For this review, use the dimensioned drawing (mm, ordinates from the lowest corner) and the shaded views. A direction names the side the tool comes from. Give positions to 0.01 mm unless a question says otherwise; leave off trailing zeros. Loops run counter-clockwise (first coordinate to the right, second up) from the corner with the lowest first, then second, coordinate; pieces in that order, holes last. Notation, with made-up numbers: (82, 5.25) - (110, 5.25) arc R24 ccw to (110, 20.25) - close; hole circle Ø3 at (45.25, 62.5). An arc over 180 degrees is marked (long way). Write each question's results on one line, items separated by ' | '.
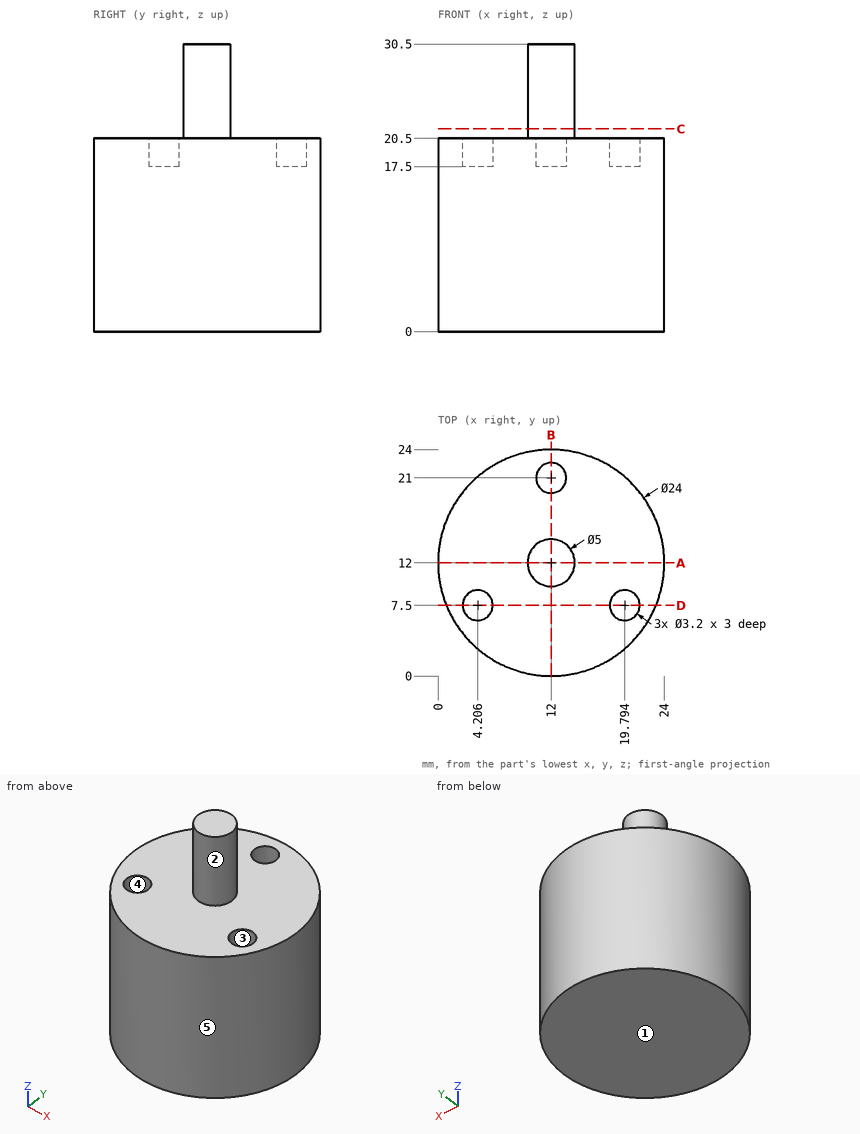
Item 1: We need section B-B on x = 12. Give the boundary of the cut face in (y, z).
Output values:
outline: (0, 0) - (24, 0) - (24, 20.5) - (22.6, 20.5) - (22.6, 17.5) - (19.4, 17.5) - (19.4, 20.5) - (14.5, 20.5) - (14.5, 30.5) - (9.5, 30.5) - (9.5, 20.5) - (0, 20.5) - close
Item 2: Wall thickness on probe 1 along Y at (x, z) = (12, 19.6); probe 2 along Z at (x, y) = (14.5, 7); probe 3 along Y at (x, z) = (6.25, 14): over which ranges is each line inside the solid? List them lowest first.
Output values:
probe 1: y = 0 to 19.4, 22.6 to 24 | probe 2: z = 0 to 20.5 | probe 3: y = 1.47 to 22.53
Item 3: Draft analysis for pull direction Y (two halves, no side actions). For the marked faces 1, 2 and 3, state which applies: +Y half, -Y half, draft (parallel to the pull), parting line (faces both ways), or undercut.
Output values:
face 1: draft | face 2: parting line | face 3: undercut
Item 4: We need section C-C on z = 21.5. Give the boundary of the cut face in (x, y).
Output values:
outline: circle Ø5 at (12, 12)
Item 5: We need section D-D on y = 7.5. Give the boundary of the cut face in (x, z).
Output values:
outline: (0.88, 0) - (23.12, 0) - (23.12, 20.5) - (21.39, 20.5) - (21.39, 17.5) - (18.19, 17.5) - (18.19, 20.5) - (5.81, 20.5) - (5.81, 17.5) - (2.61, 17.5) - (2.61, 20.5) - (0.88, 20.5) - close
Item 6: Tool access review of the marked faces 4 and 5: name each direction out of +Z, -Z, +X, -X, +Y, -Y from which nothing blocks a thin tool from reaching the whole face with its end or side.
Output values:
face 4: +Z | face 5: +Z, -Z
Item 7: We need section A-A on y = 12. Give the boundary of the cut face in (x, z).
Output values:
outline: (0, 0) - (24, 0) - (24, 20.5) - (14.5, 20.5) - (14.5, 30.5) - (9.5, 30.5) - (9.5, 20.5) - (0, 20.5) - close
Item 8: Clearance check with flat-ended pins moving along their axes: P1, Ø3.5, axis at x = 20, y = 6.5, coming from the +Z side; P2, Ø10, axis at y = 21.5, z = 11, coming from the -X side; P3, Ø1, axis at x = 12, y = 21, coming from the +Z side. State where each tip first meets the part, or that it passes through.
Output values:
P1: stops at z = 20.5 | P2: stops at x = 0.88 | P3: stops at z = 17.5
